from build123d import *

# Parameters (mm, degrees)
F1_R = 8.04
F3_R = 7.99
F5_R = 1
F6_T = -0.84


with BuildPart() as f4:
    # F1 (on Top) → F4 section 0
    with BuildSketch(Plane.XY):
        Circle(F1_R)
    # F3 (on offset) → F4 section 1
    with BuildSketch(Plane.XY.offset(40)):
        Circle(F3_R)
    loft()

    # F5
    f5_edges = [f4.edges().sort_by_distance(p)[0] for p in [
        (-7.99, 0, 40),
    ]]
    fillet(f5_edges, radius=F5_R)

    # F6
    f6_openings = [f4.faces().sort_by_distance(p)[0] for p in [
        (0, 0, 0),
    ]]
    offset(amount=F6_T, openings=f6_openings, kind=Kind.INTERSECTION)


solid = f4.part
Can you work these out from the model? Positions are in its coordinate system, mm. Give positions to 0.01 mm unless a question says otherwise; leave off trailing zeros. Loops run counter-clockwise (first coordinate to the right, second up) from the corner with the lowest first, then second, coordinate; pieces in that order, holes last. Notation, with made-up numbers: M -22,50.5 L 21,50.5 A22 cw 21,78.5 Z; hole C 3,3.5 d8. An arc over 180 degrees is marked long. One line per item, written item: value.
1) Thinking about a two-plate mould opening in Y: for faces 1 (the face through (-6.36, -4.88, 19.77)), 2 (the face through (0, 0, 40)), 3 (the face through (-0.934, 7.114, 19.773)), 4 (the face through (0, 0, 39.16)), which applies, +Y half, -Y half, draft (parallel to the pull), parting line (faces both ways), or undercut?
Geometry check:
face 1: parting line
face 2: draft
face 3: undercut
face 4: undercut
2) Please list where these lines run through material, in increasing order: line 1 (Y direction, x = 0.5, z = 18.5); line 2 (X direction, y = -1.5, z = 13.5); line 3 (Z direction, x = 1.25, y = -4.75).
Geometry check:
line 1: y = -8 to -7.16, 7.16 to 8
line 2: x = -7.88 to -7.02, 7.02 to 7.88
line 3: z = 39.16 to 40
3) Imagine slicing it at B-B on z = 13. Write out the boundary of the cut face in (x, y).
Geometry check:
outline: C 0,0 d16.05; hole C 0,0 d14.37
4) I'm going to push flat-ended pins straight in: pin 1 (2 mm diameter, centred on y = -4.5, z = 29.5, fed in from -X); pin 2 (1.5 mm diameter, centred on x = -2.5, z = 10.5, fed in from +Y); pin 3 (5 mm diameter, centred on y = 4, z = 27.5, fed in from -X). Where does each tip first touch, or does it pass through?
Geometry check:
pin 1: stops at x = -7.2
pin 2: stops at y = 7.83
pin 3: stops at x = -7.86
5) Imagine slicing it at A-A on z = 34. Write out the boundary of the cut face in (x, y) (1 decimal), and give its area (3 significant figures).
Geometry check:
outline: C 0,0 d16; hole C 0,0 d14.3
area: 40.0 mm²
